```python
from build123d import *

# Parameters (mm, degrees)
CROQUIS1_W              = 40
CROQUIS1_H              = 40
SALIENTE_EXTRUIR1_DEPTH = 1.5
CROQUIS2_R              = 7
CORTAR_EXTRUIR1_DEPTH   = 1.5
CROQUIS3_W              = 30
CROQUIS3_H              = 36
CROQUIS3_W_2            = 25
CROQUIS3_H_2            = 30
SALIENTE_EXTRUIR2_DEPTH = 4.5
CROQUIS4_R              = 14.5
CROQUIS4_R_2            = 9.5
SALIENTE_EXTRUIR3_DEPTH = 7.5
REDONDEO1_R             = 2


with BuildPart() as part:
    # Croquis1 → Saliente-Extruir1 (new body)
    with BuildSketch(Plane(origin=(0, 0, 0), x_dir=(1, 0, 0), z_dir=(0, 1, 0))):
        Rectangle(CROQUIS1_W, CROQUIS1_H)
    extrude(amount=SALIENTE_EXTRUIR1_DEPTH)

    # Croquis2 → Cortar-Extruir1 (cut)
    with BuildSketch(Plane(origin=(0, 1.5, 0), x_dir=(1, 0, 0), z_dir=(0, 1, 0))):
        with Locations((0, 2)):
            Circle(CROQUIS2_R)
    extrude(amount=-CORTAR_EXTRUIR1_DEPTH, mode=Mode.SUBTRACT)

    # Croquis3 → Saliente-Extruir2 (add)
    with BuildSketch(Plane(origin=(0, 1.5, 0), x_dir=(1, 0, 0), z_dir=(0, 1, 0))):
        Rectangle(CROQUIS3_W, CROQUIS3_H)
        Rectangle(CROQUIS3_W_2, CROQUIS3_H_2, mode=Mode.SUBTRACT)
    extrude(amount=SALIENTE_EXTRUIR2_DEPTH)

    # Croquis4 → Saliente-Extruir3 (add)
    with BuildSketch(Plane.XZ):
        with Locations((0, -2)):
            Circle(CROQUIS4_R)
        with Locations((0, -2)):
            Circle(CROQUIS4_R_2, mode=Mode.SUBTRACT)
    extrude(amount=SALIENTE_EXTRUIR3_DEPTH)

    # Redondeo1
    redondeo1_edges = [part.edges().sort_by_distance(p)[0] for p in [
        (-14.5, -7.5, -2),
        (-9.5, -7.5, -2),
    ]]
    fillet(redondeo1_edges, radius=REDONDEO1_R)


solid = part.part
```
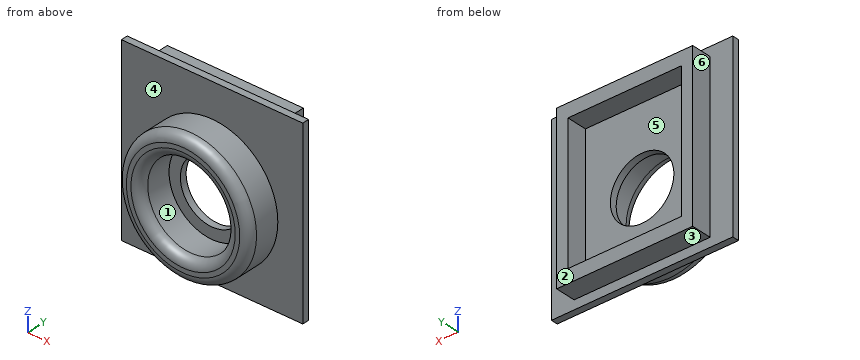
Check sheet for the modelled part. Datum: model origin and axes. Units: mm. Face numbers are marked on the shaded views. A direction names the side the tool comes from. Round coordinates to 2 decimals unless told otherwise and drop trailing zeros. Write each loop counter-clockwise with the first axis right and the second up, starting at its lowest first coordinate (ties: lowest second). Pieces come first, ordered by that corner, then holes. Notation, with made-up numbers: (-6.5, -10) -> (34.5, -10) arc R27 cw to (34.5, 11) -> close; hole circle Ø4 at (4, 22). An arc over 180 degrees is marked (long way). Put each result on its own line as item: value.
(1) Sectioned sample at B-B (x = 0). Enter the section's corners in (y, z), plus the area to 3 significant figures.
Values found:
outline: (-7.5, -14.5) arc R2 ccw to (-5.5, -16.5) -> (0, -16.5) -> (0, -20) -> (1.5, -20) -> (1.5, -18) -> (6, -18) -> (6, -15) -> (1.5, -15) -> (1.5, -9) -> (0, -9) -> (0, -11.5) -> (-5.5, -11.5) arc R2 ccw to (-7.5, -13.5) -> close; (-7.5, 9.5) arc R2 ccw to (-5.5, 7.5) -> (0, 7.5) -> (0, 5) -> (1.5, 5) -> (1.5, 15) -> (6, 15) -> (6, 18) -> (1.5, 18) -> (1.5, 20) -> (0, 20) -> (0, 12.5) -> (-5.5, 12.5) arc R2 ccw to (-7.5, 10.5) -> close
area: 138 mm^2
(2) Sectioned sample at C-C (y = 3.75). Enter the section's corners in (x, z), plus the area to 3 significant figures.
Values found:
outline: (-15, -18) -> (15, -18) -> (15, 18) -> (-15, 18) -> close; hole (-12.5, -15) -> (12.5, -15) -> (12.5, 15) -> (-12.5, 15) -> close
area: 330 mm^2
(3) Sectioned sample at D-D (z = 16.5). Enter the section's corners in (x, y).
Values found:
outline: (-20, 0) -> (20, 0) -> (20, 1.5) -> (15, 1.5) -> (15, 6) -> (-15, 6) -> (-15, 1.5) -> (-20, 1.5) -> close
(4) Tool access check on the marked faces 4, 5 and 6. Record the directions out of +Z, -Z, +X, -X, +Y, -Y that give a thin tool (end or side, any length) a straight path to the whole face; none if there is none.
Values found:
face 4: -Y
face 5: +Y
face 6: +Z, -Z, -X, +Y
(5) Go/stop test with flat-tipped pins: pin 1 Ø1.3 at (x, y) = (-7.5, 4) entering from +Z; pin 2 Ø3.5 at (x, y) = (5.5, 4.5) entering from -Z; pin 3 Ø1 at (x, y) = (7.5, -4.5) entering from -Z. Record where each tip stops, or that it passes through.
Values found:
pin 1: stops at z = 18
pin 2: stops at z = -18
pin 3: stops at z = -14.7
(6) Material ranges on line 1 (X direction, y = 1.2, z = -2); line 2 (Z direction, x = 0, y = -2.7); line 3 (Z direction, x = 0, y = 0.4), recorded low to high.
Values found:
line 1: x = -20 to -7, 7 to 20
line 2: z = -16.5 to -11.5, 7.5 to 12.5
line 3: z = -20 to -9, 5 to 20
(7) Sectioned sample at A-A (z = -2). Enter the section's corners in (x, y).
Values found:
outline: (-20, 0) -> (-14.5, 0) -> (-14.5, -5.5) arc R2 ccw to (-12.5, -7.5) -> (-11.5, -7.5) arc R2 ccw to (-9.5, -5.5) -> (-9.5, 0) -> (-7, 0) -> (-7, 1.5) -> (-12.5, 1.5) -> (-12.5, 6) -> (-15, 6) -> (-15, 1.5) -> (-20, 1.5) -> close; (7, 0) -> (9.5, 0) -> (9.5, -5.5) arc R2 ccw to (11.5, -7.5) -> (12.5, -7.5) arc R2 ccw to (14.5, -5.5) -> (14.5, 0) -> (20, 0) -> (20, 1.5) -> (15, 1.5) -> (15, 6) -> (12.5, 6) -> (12.5, 1.5) -> (7, 1.5) -> close
(8) Mould release check, pull along Z, two halves, no side actions. Record for the marked faces 1, 2 and 3: released by +Z, released by -Z, zero draft, split by the parting line, or undercut.
Values found:
face 1: undercut
face 2: zero draft
face 3: released by -Z
